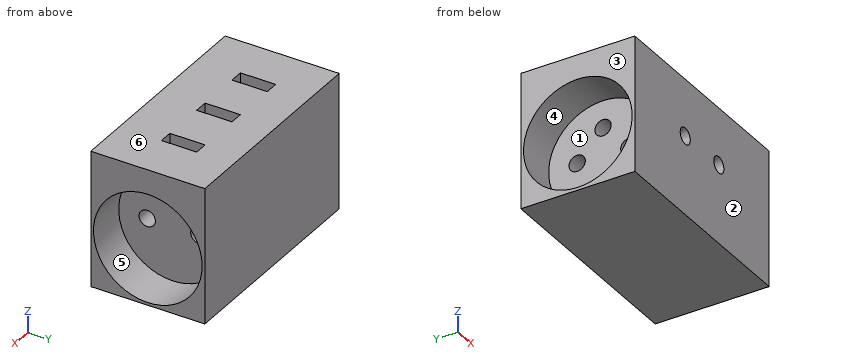
from build123d import *

# Parameters (mm, degrees)
F0_W      = 80
F0_H      = 42
F1_DEPTH  = 50
F2_W      = 5
F2_H      = 13
F3_DEPTH  = 12
F4_W      = 5
F4_H      = 13
F5_DEPTH  = 12
F6_W      = 5
F6_H      = 13
F7_DEPTH  = 12
F8_R      = 20
F9_DEPTH  = 15
F10_R     = 3
F11_DEPTH = 20
F12_R     = 3
F13_DEPTH = 20
F14_R     = 3
F15_DEPTH = 20
F16_R     = 20
F17_DEPTH = 15
F18_R     = 3
F19_DEPTH = 20
F20_R     = 3
F21_DEPTH = 20
F22_R     = 3
F23_DEPTH = 20
F24_R     = 3
F25_DEPTH = 15
F26_R     = 3
F27_DEPTH = 15


with BuildPart() as f1:
    # F0 (on Top) → F1 (new body)
    with BuildSketch(Plane.XY):
        with Locations((42.418869, -21)):
            Rectangle(F0_W, F0_H)
    extrude(amount=F1_DEPTH)

    # F2 (on face) → F3 (cut)
    with BuildSketch(Plane.XY.offset(50)):
        with Locations((20.918869, -20)):
            Rectangle(F2_W, F2_H)
    extrude(amount=-F3_DEPTH, mode=Mode.SUBTRACT)

    # F4 (on face) → F5 (cut)
    with BuildSketch(Plane.XY.offset(50)):
        with Locations((41.918869, -20)):
            Rectangle(F4_W, F4_H)
    extrude(amount=-F5_DEPTH, mode=Mode.SUBTRACT)

    # F6 (on face) → F7 (cut)
    with BuildSketch(Plane.XY.offset(50)):
        with Locations((62.918869, -20)):
            Rectangle(F6_W, F6_H)
    extrude(amount=-F7_DEPTH, mode=Mode.SUBTRACT)

    # F8 (on face) → F9 (cut)
    with BuildSketch(Plane.YZ.offset(82.418869)):
        with Locations((-21, 21)):
            Circle(F8_R)
    extrude(amount=-F9_DEPTH, mode=Mode.SUBTRACT)

    # F10 (on face) → F11 (cut)
    with BuildSketch(Plane.YZ.offset(67.418869)):
        with Locations((-11.5, 21)):
            Circle(F10_R)
    extrude(amount=-F11_DEPTH, mode=Mode.SUBTRACT)

    # F12 (on face) → F13 (cut)
    with BuildSketch(Plane.YZ.offset(67.418869)):
        with Locations((-30.5, 21)):
            Circle(F12_R)
    extrude(amount=-F13_DEPTH, mode=Mode.SUBTRACT)

    # F14 (on face) → F15 (cut)
    with BuildSketch(Plane.YZ.offset(67.418869)):
        with Locations((-21, 31)):
            Circle(F14_R)
    extrude(amount=-F15_DEPTH, mode=Mode.SUBTRACT)

    # F16 (on face) → F17 (cut)
    with BuildSketch(Plane(origin=(2.418869, 0, 0), x_dir=(0, -1, 0), z_dir=(-1, 0, 0))):
        with Locations((21, 21)):
            Circle(F16_R)
    extrude(amount=-F17_DEPTH, mode=Mode.SUBTRACT)

    # F18 (on face) → F19 (cut)
    with BuildSketch(Plane(origin=(17.418869, 0, 0), x_dir=(0, -1, 0), z_dir=(-1, 0, 0))):
        with Locations((30.5, 21)):
            Circle(F18_R)
    extrude(amount=-F19_DEPTH, mode=Mode.SUBTRACT)

    # F20 (on face) → F21 (cut)
    with BuildSketch(Plane(origin=(17.418869, 0, 0), x_dir=(0, -1, 0), z_dir=(-1, 0, 0))):
        with Locations((11.5, 21)):
            Circle(F20_R)
    extrude(amount=-F21_DEPTH, mode=Mode.SUBTRACT)

    # F22 (on face) → F23 (cut)
    with BuildSketch(Plane(origin=(17.418869, 0, 0), x_dir=(0, -1, 0), z_dir=(-1, 0, 0))):
        with Locations((21, 31)):
            Circle(F22_R)
    extrude(amount=-F23_DEPTH, mode=Mode.SUBTRACT)

    # F24 (on face) → F25 (cut)
    with BuildSketch(Plane.XZ.offset(42)):
        with Locations((32.418869, 29)):
            Circle(F24_R)
    extrude(amount=-F25_DEPTH, mode=Mode.SUBTRACT)

    # F26 (on face) → F27 (cut)
    with BuildSketch(Plane.XZ.offset(42)):
        with Locations((52.418869, 29)):
            Circle(F26_R)
    extrude(amount=-F27_DEPTH, mode=Mode.SUBTRACT)


solid = f1.part
The listing builds one solid part. Answer for the finished solid, in the listing's coordinates (mm). Face numbers are marked on the shaded views. A direction names the side the tool comes from. Round coordinates to 2 decimals unless told otherwise and drop trailing zeros. Write each loop counter-clockwise with the first axis right and the second up, starting at its lowest first coordinate (ties: lowest second). Pieces come first, ordered by that corner, then holes. Notation, with made-up numbers: (24.5, 42.25) - (65.5, 42.25) arc R22 cw to (65.5, 79.25) - close; hole circle Ø7 at (-18, -10.5). An arc over 180 degrees is marked (long way). Use a Markdown table: item, result. Add a question column.
1. The part is cut by section C-C (x = 75.5). Write down the section's boundary in (y, z), and give its area (3 significant figures).
2. For a pull along Y with two mould halves and no side action, classify the marked faces 1, 2 and 3 as +Y half, -Y half, draft (parallel to the pull), parting line (faces both ways), or undercut.
3. The part is cut by section A-A (x = 28.5). Write down the section's boundary in (y, z), and give its area (3 significant figures).
4. A tool of negligible diameter and unlimited length cuts with its end or side. For the marked faces 4, 5 and 6, from which of +Z, -Z, +X, -X, +Y, -Y can it reach the whole face along a straight path? Write none if from no direction.
5. The part is cut by section B-B (z = 21). Write down the section's boundary in (x, y), and give its area (3 significant figures).
6. The part is cut by section D-D (y = -30.5). Write down the section's boundary in (x, z).
7. Flat-ended cylindrical pins translate along their axes: P1, Ø3, axis at y = -20.5, z = 31.5, coming from the +X side; P2, Ø1.8, axis at y = -21, z = 31.5, coming from the -X side; P3, Ø8, axis at y = -21, z = 31, coming from the -X side. Find the tip coordinate at first contact, or state that the pin passes through.
8. Consider line 1 (X direction, y = -20, z = 43.5); line 2 (Z direction, x = 23, y = -21); line 3 (Z direction, x = 75, y = -21). Determine where each line is inside the solid, lowest interval first.
Reported:
| question | item | result |
|---|---|---|
| 1 | outline | (-42, 0) - (0, 0) - (0, 50) - (-42, 50) - close; hole circle Ø40 at (-21, 21) |
| 1 | area | 843 mm^2 |
| 2 | face 1 | undercut |
| 2 | face 2 | -Y half |
| 2 | face 3 | draft |
| 3 | outline | (-42, 0) - (0, 0) - (0, 50) - (-42, 50) - close; hole circle Ø6 at (-30.5, 21); hole circle Ø6 at (-21, 31); hole circle Ø6 at (-11.5, 21) |
| 3 | area | 2,020 mm^2 |
| 4 | face 4 | -X |
| 4 | face 5 | +X |
| 4 | face 6 | +Z, +X, -X, +Y, -Y |
| 5 | outline | (2.42, -42) - (82.42, -42) - (82.42, -41) - (67.42, -41) - (67.42, -33.5) - (47.42, -33.5) - (47.42, -27.5) - (67.42, -27.5) - (67.42, -14.5) - (47.42, -14.5) - (47.42, -8.5) - (67.42, -8.5) - (67.42, -1) - (82.42, -1) - (82.42, 0) - (2.42, 0) - (2.42, -1) - (17.42, -1) - (17.42, -8.5) - (37.42, -8.5) - (37.42, -14.5) - (17.42, -14.5) - (17.42, -27.5) - (37.42, -27.5) - (37.42, -33.5) - (17.42, -33.5) - (17.42, -41) - (2.42, -41) - close |
| 5 | area | 1,680 mm^2 |
| 6 | outline | (2.42, 0) - (82.42, 0) - (82.42, 3.4) - (67.42, 3.4) - (67.42, 18) - (47.42, 18) - (47.42, 24) - (67.42, 24) - (67.42, 38.6) - (82.42, 38.6) - (82.42, 50) - (2.42, 50) - (2.42, 38.6) - (17.42, 38.6) - (17.42, 24) - (37.42, 24) - (37.42, 18) - (17.42, 18) - (17.42, 3.4) - (2.42, 3.4) - close; hole circle Ø6 at (32.42, 29); hole circle Ø6 at (52.42, 29) |
| 7 | P1 | x = 47.42 |
| 7 | P2 | x = 37.42 |
| 7 | P3 | x = 17.42 |
| 8 | line 1 | 2.42 to 18.42, 23.42 to 39.42, 44.42 to 60.42, 65.42 to 82.42 |
| 8 | line 2 | 0 to 28, 34 to 38 |
| 8 | line 3 | 0 to 1, 41 to 50 |
